from build123d import *

# Parameters (mm, degrees)
SKETCH1_W                      = 450
SKETCH1_H                      = 45.7
BOSS_EXTRUDE1_DEPTH            = 11.4
CUT_EXTRUDE1_DEPTH             = 451
SKETCH3_W                      = 10.25
SKETCH3_H                      = 23.6
CUT_EXTRUDE2_DEPTH             = 12.4
CUT_EXTRUDE3_DEPTH             = 2.27
CUT_EXTRUDE4_DEPTH             = 2.27
CUT_EXTRUDE5_DEPTH             = 2.27
CUT_EXTRUDE6_DEPTH             = 2.27
CUT_EXTRUDE7_DEPTH             = 2.27
CUT_EXTRUDE8_DEPTH             = 2.27
CUT_EXTRUDE9_DEPTH             = 2.27
CUT_EXTRUDE10_DEPTH            = 2.27
CUT_EXTRUDE11_DEPTH            = 2.27
CUT_EXTRUDE12_DEPTH            = 12.4
F_6_4_6_4_DIAMETER_HOLE1_D     = 6.4
F_6_4_6_4_DIAMETER_HOLE1_DEPTH = 11.4
F_4_6_4_6_DIAMETER_HOLE1_D     = 4.6
F_4_6_4_6_DIAMETER_HOLE1_DEPTH = 11.4
SCALE1_SCALE                   = 0.25


with BuildPart() as part:
    # Sketch1 → Boss-Extrude1 (new body)
    with BuildSketch(Plane(origin=(5.7, 0, 0), x_dir=(0, 0, -1), z_dir=(1, 0, 0))):
        with Locations((-225, 0)):
            Rectangle(SKETCH1_W, SKETCH1_H)
    extrude(amount=-BOSS_EXTRUDE1_DEPTH)

    # Sketch2 → Cut-Extrude1 (cut, through all)
    with BuildSketch(Plane.XY.offset(450)):
        Polygon((5.7, 17.85), (4.43, 17.85), (4.43, 21.58), (-4.43, 21.58), (-4.43, -21.58), (4.43, -21.58), (4.43, -17.85), (5.7, -17.85), align=None)
    extrude(amount=-CUT_EXTRUDE1_DEPTH, mode=Mode.SUBTRACT)

    # Sketch3 → Cut-Extrude2 (cut, through all)
    with BuildSketch(Plane.ZY.offset(5.7)):
        with Locations((5.125, 0)):
            Rectangle(SKETCH3_W, SKETCH3_H)
    extrude(amount=-CUT_EXTRUDE2_DEPTH, mode=Mode.SUBTRACT)

    # Sketch4 → Cut-Extrude3 (cut, through all)
    with BuildSketch(Plane(origin=(-4.43, 0, 0), x_dir=(0, 0, -1), z_dir=(1, 0, 0))):
        Polygon((-169.5, -10.25), (-169.5, -7.05), (-210.9, -7.05), (-210.9, 7.05), (-169.5, 7.05), (-169.5, 10.25), (-215.5, 10.25), (-215.5, -10.25), align=None)
    extrude(amount=-CUT_EXTRUDE3_DEPTH, mode=Mode.SUBTRACT)

    # Sketch5 → Cut-Extrude4 (cut, through all)
    with BuildSketch(Plane(origin=(-4.43, 0, 0), x_dir=(0, 0, -1), z_dir=(1, 0, 0))):
        Polygon((-119.5, -10.25), (-73.5, -10.25), (-73.5, -7.05), (-114.9, -7.05), (-114.9, 7.05), (-73.5, 7.05), (-73.5, 10.25), (-119.5, 10.25), align=None)
    extrude(amount=-CUT_EXTRUDE4_DEPTH, mode=Mode.SUBTRACT)

    # Sketch6 → Cut-Extrude5 (cut, through all)
    with BuildSketch(Plane(origin=(-4.43, 0, 0), x_dir=(0, 0, -1), z_dir=(1, 0, 0))):
        Polygon((-265.15, 7.05), (-265.15, 10.25), (-311.15, 10.25), (-311.15, -10.25), (-265.15, -10.25), (-265.15, -7.05), (-306.55, -7.05), (-306.55, 7.05), align=None)
    extrude(amount=-CUT_EXTRUDE5_DEPTH, mode=Mode.SUBTRACT)

    # Sketch7 → Cut-Extrude6 (cut, through all)
    with BuildSketch(Plane(origin=(-4.43, 0, 0), x_dir=(0, 0, -1), z_dir=(1, 0, 0))):
        with BuildLine():
            Line((-79.85, 2.3), (-84.75, 2.3))
            ThreePointArc((-84.75, 2.3), (-87.05, 0), (-84.75, -2.3))
            Line((-84.75, -2.3), (-79.85, -2.3))
            ThreePointArc((-79.85, -2.3), (-77.55, 0), (-79.85, 2.3))
        make_face()
    extrude(amount=-CUT_EXTRUDE6_DEPTH, mode=Mode.SUBTRACT)

    # Sketch8 → Cut-Extrude7 (cut, through all)
    with BuildSketch(Plane(origin=(-4.43, 0, 0), x_dir=(0, 0, -1), z_dir=(1, 0, 0))):
        with BuildLine():
            Line((-108.85, -2.3), (-103.95, -2.3))
            ThreePointArc((-103.95, -2.3), (-101.65, 0), (-103.95, 2.3))
            Line((-103.95, 2.3), (-108.85, 2.3))
            ThreePointArc((-108.85, 2.3), (-111.15, 0), (-108.85, -2.3))
        make_face()
    extrude(amount=-CUT_EXTRUDE7_DEPTH, mode=Mode.SUBTRACT)

    # Sketch9 → Cut-Extrude8 (cut, through all)
    with BuildSketch(Plane(origin=(-4.43, 0, 0), x_dir=(0, 0, -1), z_dir=(1, 0, 0))):
        with BuildLine():
            Line((-387.25, 2.3), (-392.15, 2.3))
            ThreePointArc((-392.15, 2.3), (-394.45, 0), (-392.15, -2.3))
            Line((-392.15, -2.3), (-387.25, -2.3))
            ThreePointArc((-387.25, -2.3), (-384.95, 0), (-387.25, 2.3))
        make_face()
    extrude(amount=-CUT_EXTRUDE8_DEPTH, mode=Mode.SUBTRACT)

    # Sketch10 → Cut-Extrude9 (cut, through all)
    with BuildSketch(Plane(origin=(-4.43, 0, 0), x_dir=(0, 0, -1), z_dir=(1, 0, 0))):
        with BuildLine():
            Line((-199.95, 2.3), (-204.85, 2.3))
            ThreePointArc((-204.85, 2.3), (-207.15, 0), (-204.85, -2.3))
            Line((-204.85, -2.3), (-199.95, -2.3))
            ThreePointArc((-199.95, -2.3), (-197.65, 0), (-199.95, 2.3))
        make_face()
    extrude(amount=-CUT_EXTRUDE9_DEPTH, mode=Mode.SUBTRACT)

    # Sketch11 → Cut-Extrude10 (cut, through all)
    with BuildSketch(Plane(origin=(-4.43, 0, 0), x_dir=(0, 0, -1), z_dir=(1, 0, 0))):
        with BuildLine():
            Line((-295.95, 2.3), (-300.85, 2.3))
            ThreePointArc((-300.85, 2.3), (-303.15, 0), (-300.85, -2.3))
            Line((-300.85, -2.3), (-295.95, -2.3))
            ThreePointArc((-295.95, -2.3), (-293.65, 0), (-295.95, 2.3))
        make_face()
    extrude(amount=-CUT_EXTRUDE10_DEPTH, mode=Mode.SUBTRACT)

    # Sketch12 → Cut-Extrude11 (cut, through all)
    with BuildSketch(Plane(origin=(-4.43, 0, 0), x_dir=(0, 0, -1), z_dir=(1, 0, 0))):
        with BuildLine():
            Line((-271.85, 2.3), (-276.75, 2.3))
            ThreePointArc((-276.75, 2.3), (-279.05, 0), (-276.75, -2.3))
            Line((-276.75, -2.3), (-271.85, -2.3))
            ThreePointArc((-271.85, -2.3), (-269.55, 0), (-271.85, 2.3))
        make_face()
    extrude(amount=-CUT_EXTRUDE11_DEPTH, mode=Mode.SUBTRACT)

    # Sketch13 → Cut-Extrude12 (cut, through all)
    with BuildSketch(Plane.ZY.offset(5.7)):
        Polygon((434, -7.15), (409.2, -7.15), (409.2, 7.15), (434, 7.15), (434, 10.25), (379.65, 10.25), (379.65, 7.15), (406.9, 7.15), (406.9, -7.15), (379.65, -7.15), (379.65, -10.25), (434, -10.25), align=None)
    extrude(amount=-CUT_EXTRUDE12_DEPTH, mode=Mode.SUBTRACT)

    # Ø6.4 (6.4) Diameter Hole1
    with Locations(Plane.ZY.offset(5.7)):
        with Locations((415, 0), (287, 0), (191, 0), (95, 0)):
            Hole(F_6_4_6_4_DIAMETER_HOLE1_D / 2, depth=F_6_4_6_4_DIAMETER_HOLE1_DEPTH)

    # Ø4.6 (4.6) Diameter Hole1
    with Locations(Plane.ZY.offset(5.7)):
        with Locations((424, 0), (402.4, 0), (178.3, 0)):
            Hole(F_4_6_4_6_DIAMETER_HOLE1_D / 2, depth=F_4_6_4_6_DIAMETER_HOLE1_DEPTH)


with BuildPart() as part_1:
    # Scale1: scaled about (-2.285927212, 0, 225.277222982)
    add(part.part.scale(SCALE1_SCALE).moved(Location((-1.714445409, 0, 168.957917237))))


solid = part_1.part
Verification items for the finished model (mm, model axes). A direction names the side the tool comes from. Coordinates: 2 decimals unless noted, no trailing zeros. Answer as a JSON object with one key per item and string values. Group by question number.
Item 1: Mould release check, pull along X, two halves, no side actions. Record for faces 3 (the flat face through (-2, -5.395, 226)), 4 (the flat face through (-2.974, -0.027, 281.458)), 5 (the flat face through (-3.139, 0, 226)): +X half, -X half, draft (parallel to the pull), parting line (faces both ways), or undercut.
Item 2: Tool access check on faces 1 (the flat face through (-2, 5.712, 226)), 2 (the flat face through (-2, 5.395, 226)). Record the directions out of +Z, -Z, +X, -X, +Y, -Y that give a thin tool (end or side, any length) a straight path to the whole face; none if there is none.
Item 3: Scan lines: probe 1 along Y at (x, z) = (-1.2, 191) (1 decimal); probe 2 along X at (y, z) = (5, 177.5); probe 3 along Y at (x, z) = (-0.55, 214). Record each from-to range of solid material in increasing order.
Evaluation:
{
 "1": {"face 3": "undercut", "face 4": "draft", "face 5": "-X half"},
 "2": {"face 1": "+Z, -Z, +X, -X, +Y", "face 2": "+Z, -Z"},
 "3": {"probe 1": "y = -5.7 to -5.4, 5.4 to 5.7", "probe 2": "x = -3.14 to -2.82, -0.61 to -0.29", "probe 3": "y = -5.71 to -4.46, 4.46 to 5.71"}
}
